Here's the drawing with two shaded views (mm, measured from the low corner). I have some questions. A direction names the side the tool comes from. Coordinates: 2 decimals unless noted, no trailing zeros. Write each loop counter-clockwise with the first axis right and the second up, starting at its lowest first coordinate (ties: lowest second). Pieces come first, ordered by that corner, then holes.
Item 1: If we section it at B-B (z = 12.5): Please give me the cut outline in (x, y), then the cut area to 3 significant figures.
Item 2: If I drill on line 1 (Y direction, x = 133, z = 11.5); line 2 (Z direction, x = 90.5, y = 13.5), over which ranges is the centre line in solid material (lowest first)?
Item 3: For the marked faces 1 and 2, which set-ups out of +Z, -Z, +X, -X, +Y, -Y let a thin tool reach every point of the face, with its end or its side?
Item 4: I'm going to push a flat-ended pin straight in: pin 1 Ø6 at (x, z) = (283.5, 10.5) entering from -Y. Where does the tip first touch, or does it pass through?
Item 5: If we section it at C-C (y = 46.5): Please give me the cut outline in (x, z).
Item 6: If we section it at A-A (x = 215): Please give me the cut outline in (y, z), then the cut area to 3 significant figures.
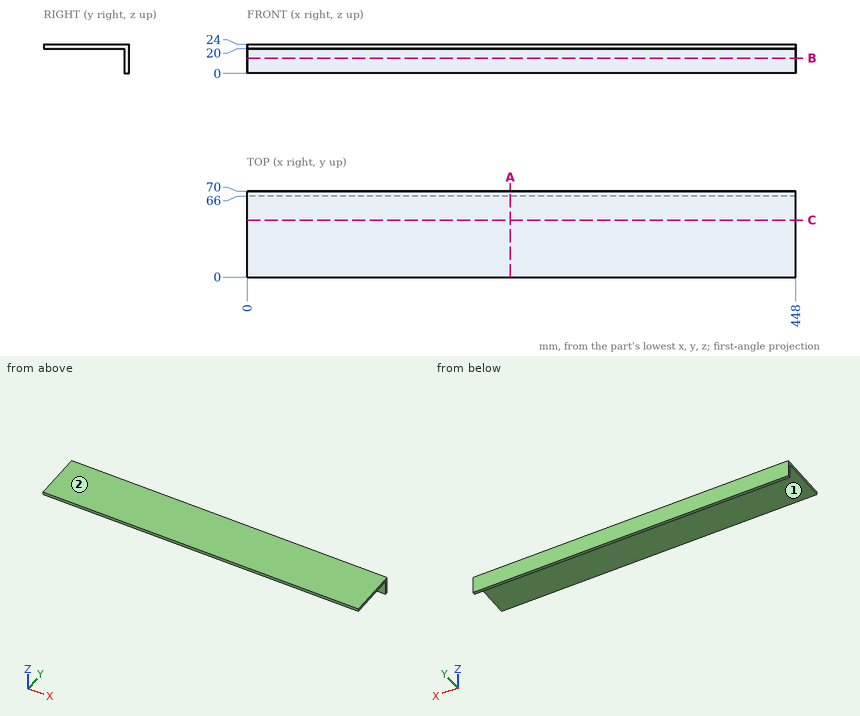
Answer list:
1. outline: (0, 66) - (448, 66) - (448, 70) - (0, 70) - close
1. area: 1,790 mm2
2. line 1: y = 66 to 70
2. line 2: z = 20 to 24
3. face 1: -Z, +X, -X, -Y
3. face 2: +Z, +X, -X, +Y, -Y
4. pin 1: stops at y = 66
5. outline: (0, 20) - (448, 20) - (448, 24) - (0, 24) - close
6. outline: (0, 20) - (66, 20) - (66, 0) - (70, 0) - (70, 24) - (0, 24) - close
6. area: 360 mm2
